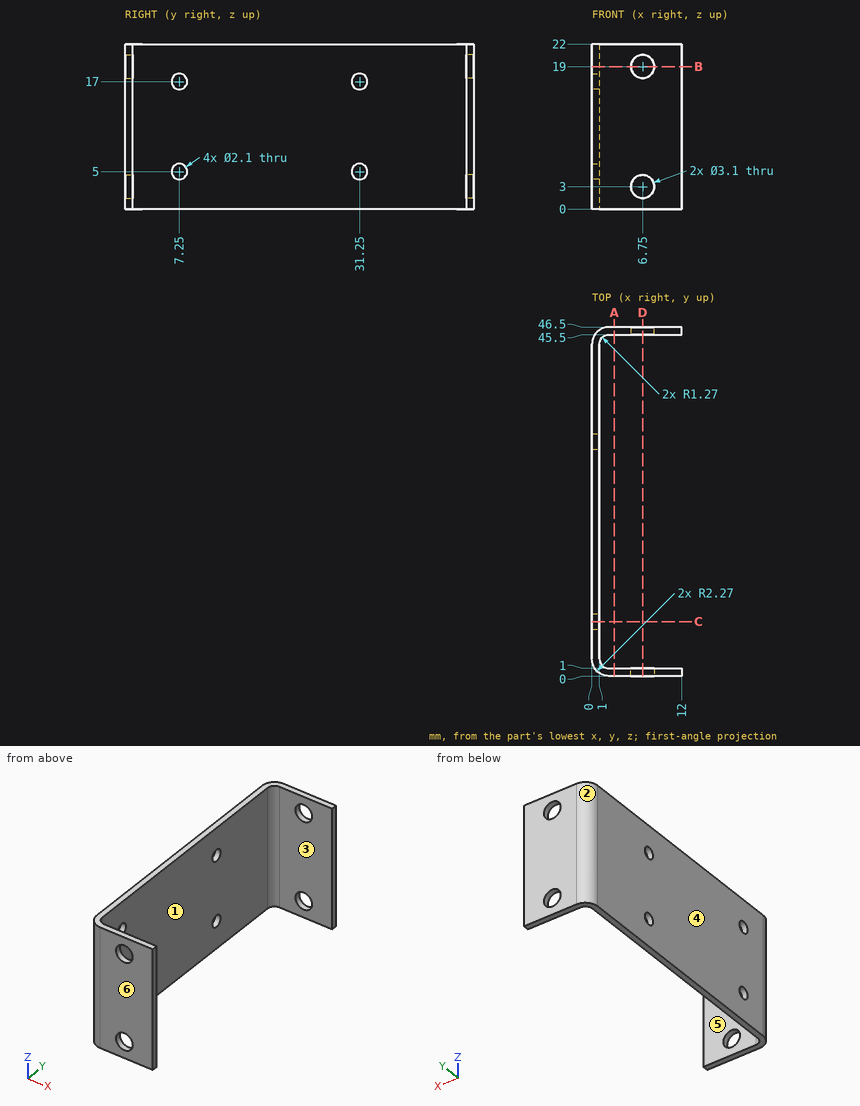
Can you work these out from the drawing? Everything is in mm from the part's minimum corner. A direction names the side the tool comes from. Round coordinates to 2 decimals unless told otherwise and drop trailing zeros. Order: outer loops, then holes, each group sorted by start corner. A loop starts at its lowest first (then second) coordinate and runs counter-clockwise, first axis right, second up. Notation, with made-up numbers: M 82,-35.75 L 92,-35.75 A6 cw 92,-27.75 Z; hole C 76.25,20 d10. An arc over 180 degrees is marked long. One line per question, with ' | ' between items.
1) For pin 1 Ø2.5 at (x, z) = (6.75, 19) entering from -Y; pin 2 Ø2.5 at (y, z) = (7.25, 5) entering from +X, each with a flat end and sliding along its axis, tell me the tip position at first contact or that it passes through.
Working result:
pin 1: through | pin 2: x = 1
2) I want a section at B-B, the plane z = 19. Write out the boundary of the cut face in (x, y), then the cut area to 3 significant figures.
Working result:
outline: M 0,2.27 A2.27 ccw 2.27,0 L 5.2,0 L 5.2,1 L 2.27,1 A1.27 cw 1,2.27 L 1,44.23 A1.27 cw 2.27,45.5 L 5.2,45.5 L 5.2,46.5 L 2.27,46.5 A2.27 ccw 0,44.23 Z; M 8.3,0 L 12,0 L 12,1 L 8.3,1 Z; M 8.3,45.5 L 12,45.5 L 12,46.5 L 8.3,46.5 Z | area: 60.8 mm²
3) For the marked faces 5 and 6, which set-ups out of +Z, -Z, +X, -X, +Y, -Y let a thin tool reach every point of the face, with its end or its side?
Working result:
face 5: +Z, -Z, +X | face 6: +Z, -Z, +X, -X, -Y
4) I need wall thicknesses on line 1 along Z through (x, y) = (6.75, 46); line 2 along Y through (x, z) = (6.75, 15); line 3 along Y through (x, z) = (0.35, 5). Which ranges of each line are inside material? Lowest first, please.
Working result:
line 1: 0 to 1.45, 4.55 to 17.45, 20.55 to 22 | line 2: 0 to 1, 45.5 to 46.5 | line 3: 1.06 to 6.2, 8.3 to 30.2, 32.3 to 45.44
5) I want a section at C-C, the plane y = 7.25. Write out the boundary of the cut face in (x, z), then the cut area to 3 significant figures.
Working result:
outline: M 0,0 L 1,0 L 1,3.95 L 0,3.95 Z; M 0,6.05 L 1,6.05 L 1,15.95 L 0,15.95 Z; M 0,18.05 L 1,18.05 L 1,22 L 0,22 Z | area: 17.8 mm²
6) I want a section at A-A, the plane x = 3. Write out the boundary of the cut face in (y, z), then the cut area to 3 significant figures.
Working result:
outline: M 0,0 L 1,0 L 1,22 L 0,22 Z; M 45.5,0 L 46.5,0 L 46.5,22 L 45.5,22 Z | area: 44.0 mm²
7) I want a section at D-D, the plane x = 6.75. Write out the boundary of the cut face in (y, z).
Working result:
outline: M 0,0 L 1,0 L 1,1.45 L 0,1.45 Z; M 0,4.55 L 1,4.55 L 1,17.45 L 0,17.45 Z; M 0,20.55 L 1,20.55 L 1,22 L 0,22 Z; M 45.5,0 L 46.5,0 L 46.5,1.45 L 45.5,1.45 Z; M 45.5,4.55 L 46.5,4.55 L 46.5,17.45 L 45.5,17.45 Z; M 45.5,20.55 L 46.5,20.55 L 46.5,22 L 45.5,22 Z
8) If we mould it in two halves opening along Y, with no side actions, what happens to the marked faces 1, 2, 3 and 4? For each: +Y half, -Y half, draft (parallel to the pull), parting line (faces both ways), or undercut.
Working result:
face 1: undercut | face 2: +Y half | face 3: undercut | face 4: draft
